Geometry: final body of the model. Coordinates: model frame, mm. Round coordinates to 2 decimals unless told otherwise and drop trailing zeros. Loops run counter-clockwise (first coordinate to the right, second up) from the corner with the lowest first, then second, coordinate; pieces in that order, holes last. Notation, with made-up numbers: (53, 11) - (88, 11) arc R10 cw to (88, 16) - close; hole circle Ø7 at (81, -25). An arc over 180 degrees is marked (long way). Return JSON: item names as keys, results as strings. Group by question number.
1. Section C-C on z = 31. Return loops of the section in (x, y), and give its area (3 significant figures).
2. Section A-A on x = 0.5. Return loops of the section in (y, z).
3. Section B-B on z = -96. Return loops of the section in (x, y), and give its area (3 significant figures).
4. First-contact query: pin 1 Ø1 at (x, y) = (1.5, 54.5) entering from -Z; pin 2 Ø1.5 at (x, z) = (1.5, 118.5) entering from +Y; pin 3 Ø1.5 at (x, z) = (1.5, -182) entering from +Y. Flat tips, straight axial feed; report the tip coordinate or a pass-through.
5. Material intervals for probe 1 along Z at (x, y) = (1.95, 30); probe 2 along Z at (x, y) = (2.4, 39.5); probe 3 along Y at (x, z) = (1.35, -91.5), sorted ascending.
from build123d import *

# Parameters (mm, degrees)
BOSS_EXTRUDE1_DEPTH      = 3
CUT_EXTRUDE2_DEPTH       = 295.638673234
CUT_EXTRUDE2_DEPTH_BACK  = 3
CUT_EXTRUDE6_DEPTH       = 295.638673234
CUT_EXTRUDE6_DEPTH_BACK  = 3
CUT_EXTRUDE11_DEPTH      = 295.638673234
CUT_EXTRUDE11_DEPTH_BACK = 3
CUT_EXTRUDE12_DEPTH      = 295.638673234
CUT_EXTRUDE12_DEPTH_BACK = 3
SKETCH9_W                = 3
SKETCH9_H                = 30
CUT_EXTRUDE13_DEPTH      = 3


with BuildPart() as part:
    # Sketch1 → Boss-Extrude1 (new body)
    with BuildSketch(Plane(origin=(0, 0, 0), x_dir=(0, 0, -1), z_dir=(1, 0, 0))):
        Polygon((286.144320394, 0.17389594), (286.144320394, 70.17389594), (-16.855679606, 70.17389594), (-116.855679606, 40.17389594), (-119.855679606, 40.17389594), (-119.855679606, 0.17389594), align=None)
    extrude(amount=BOSS_EXTRUDE1_DEPTH)

    # Sketch5 → Cut-Extrude2 (cut, two sides: drawn at the far end of the back side and taken through both)
    with BuildSketch(Plane(origin=(3, 0, 0), x_dir=(0, 0, -1), z_dir=(1, 0, 0)).offset(-CUT_EXTRUDE2_DEPTH_BACK)):
        Polygon((1115.56118622, 55.17389594), (286.144320394, 55.17389594), (283.144320394, 55.17389594), (283.144320394, 15.17389594), (286.144320394, 15.17389594), (1115.56118622, 15.17389594), (2774.394917872, 15.17389594), (2774.394917872, 55.17389594), align=None)
    extrude(amount=CUT_EXTRUDE2_DEPTH + CUT_EXTRUDE2_DEPTH_BACK, mode=Mode.SUBTRACT)

    # Sketch6 → Cut-Extrude6 (cut, two sides: drawn at the far end of the back side and taken through both)
    with BuildSketch(Plane(origin=(3, 0, 0), x_dir=(0, 0, -1), z_dir=(1, 0, 0)).offset(-CUT_EXTRUDE6_DEPTH_BACK)):
        Polygon((253.144320394, 839.196952243), (253.144320394, 70.17389594), (253.144320394, 67.17389594), (13.144320394, 67.17389594), (13.144320394, 70.17389594), (13.144320394, 839.196952243), (13.144320394, 2377.24306485), (253.144320394, 2377.24306485), align=None)
    extrude(amount=CUT_EXTRUDE6_DEPTH + CUT_EXTRUDE6_DEPTH_BACK, mode=Mode.SUBTRACT)

    # Sketch7 → Cut-Extrude11 (cut, two sides: drawn at the far end of the back side and taken through both)
    with BuildSketch(Plane(origin=(3, 0, 0), x_dir=(0, 0, -1), z_dir=(1, 0, 0)).offset(-CUT_EXTRUDE11_DEPTH_BACK)):
        Polygon((-264.146282978, 799.817128167), (-42.908554564, 62.358033452), (-42.046510907, 59.484554597), (-89.937825168, 45.117160318), (-90.799868825, 47.990639174), (-312.037597239, 785.449733889), (-754.513054068, 2260.367923318), (-706.621739807, 2274.735317597), align=None)
    extrude(amount=CUT_EXTRUDE11_DEPTH + CUT_EXTRUDE11_DEPTH_BACK, mode=Mode.SUBTRACT)

    # Sketch8 → Cut-Extrude12 (cut, two sides: drawn at the far end of the back side and taken through both)
    with BuildSketch(Plane(origin=(3, 0, 0), x_dir=(0, 0, -1), z_dir=(1, 0, 0)).offset(-CUT_EXTRUDE12_DEPTH_BACK)):
        Polygon((-950.674782697, 30.17389594), (-119.855679606, 30.17389594), (-116.855679606, 30.17389594), (-116.855679606, 10.17389594), (-119.855679606, 10.17389594), (-950.674782697, 10.17389594), (-2612.31298888, 10.17389594), (-2612.31298888, 30.17389594), align=None)
    extrude(amount=CUT_EXTRUDE12_DEPTH + CUT_EXTRUDE12_DEPTH_BACK, mode=Mode.SUBTRACT)

    # Sketch9 → Cut-Extrude13 (cut)
    with BuildSketch(Plane(origin=(3, 0, 0), x_dir=(0, 0, -1), z_dir=(1, 0, 0))):
        with Locations((-15.355679606, 35.17389594)):
            Rectangle(SKETCH9_W, SKETCH9_H)
    extrude(amount=-CUT_EXTRUDE13_DEPTH, mode=Mode.SUBTRACT)


solid = part.part
Taken from the geometry:
{
 "1": {"outline": "(0, 0.17) - (3, 0.17) - (3, 65.93) - (0, 65.93) - close", "area": "197 mm2"},
 "2": {"outline": "(0.17, -286.14) - (15.17, -286.14) - (15.17, -283.14) - (55.17, -283.14) - (55.17, -286.14) - (70.17, -286.14) - (70.17, -253.14) - (67.17, -253.14) - (67.17, -13.14) - (70.17, -13.14) - (70.17, 16.86) - (62.36, 42.91) - (59.48, 42.05) - (45.12, 89.94) - (47.99, 90.8) - (40.17, 116.86) - (40.17, 119.86) - (30.17, 119.86) - (30.17, 116.86) - (10.17, 116.86) - (10.17, 119.86) - (0.17, 119.86) - close; hole (20.17, 13.86) - (50.17, 13.86) - (50.17, 16.86) - (20.17, 16.86) - close"},
 "3": {"outline": "(0, 0.17) - (3, 0.17) - (3, 67.17) - (0, 67.17) - close", "area": "201 mm2"},
 "4": {"pin 1": "z = -283.14", "pin 2": "y = 40.17", "pin 3": "y = 67.17"},
 "5": {"probe 1": "-283.14 to 13.86, 16.86 to 116.86", "probe 2": "-283.14 to 13.86, 16.86 to 119.86", "probe 3": "0.17 to 67.17"}
}
